The listing builds one solid part. Answer for the finished solid, in the listing's coordinates (mm). A direction names the side the tool comes from. Give positions to 0.01 mm unless a question says otherwise; leave off trailing zeros. Order: outer loops, then holes, each group sorted by start corner. A loop starts at its lowest first (then second) coordinate and runs counter-clockwise, first axis right, second up. Notation, with made-up numbers: (-36, 57) -> (17, 57) arc R28 cw to (17, 75) -> close; hole circle Ø1 at (79, -20.5). An arc over 180 degrees is marked (long way). Answer as a JSON object with one key per item and string values. Group by question number.
```python
from build123d import *

# Parameters (mm, degrees)
F1_DEPTH = 8.89


with BuildPart() as f1:
    # F0 (on Front) → F1 (new body)
    with BuildSketch(Plane.XZ):
        with BuildLine():
            Line((-102.723063, 1.27), (-102.723063, 0))
            Line((-102.723063, 0), (-77.323063, 0))
            Line((-77.323063, 0), (-77.323063, 1.27))
            ThreePointArc((-77.323063, 1.27), (-77.695037, 2.168026), (-78.593063, 2.54))
            Line((-78.593063, 2.54), (-80.879063, 2.54))
            ThreePointArc((-80.879063, 2.54), (-81.058668, 2.614395), (-81.133063, 2.794))
            Line((-81.133063, 2.794), (-81.133063, 5.08))
            ThreePointArc((-81.133063, 5.08), (-81.505037, 5.978026), (-82.403063, 6.35))
            Line((-82.403063, 6.35), (-97.643063, 6.35))
            ThreePointArc((-97.643063, 6.35), (-98.541089, 5.978026), (-98.913063, 5.08))
            Line((-98.913063, 5.08), (-98.913063, 4.318))
            ThreePointArc((-98.913063, 4.318), (-98.541089, 3.419974), (-97.643063, 3.048))
            Line((-97.643063, 3.048), (-95.357063, 3.048))
            ThreePointArc((-95.357063, 3.048), (-95.177458, 3.122395), (-95.103063, 3.302))
            Line((-95.103063, 3.302), (-95.103063, 3.556))
            ThreePointArc((-95.103063, 3.556), (-95.028668, 3.735605), (-94.849063, 3.81))
            Line((-94.849063, 3.81), (-85.197063, 3.81))
            ThreePointArc((-85.197063, 3.81), (-85.017458, 3.735605), (-84.943063, 3.556))
            Line((-84.943063, 3.556), (-84.943063, 2.794))
            ThreePointArc((-84.943063, 2.794), (-85.017458, 2.614395), (-85.197063, 2.54))
            Line((-85.197063, 2.54), (-101.453063, 2.54))
            ThreePointArc((-101.453063, 2.54), (-102.351089, 2.168026), (-102.723063, 1.27))
        make_face()
    extrude(amount=F1_DEPTH)


solid = f1.part
```
(1) Find the intervals of material crossed by line 1 along Z through (x, y) = (-97.75, -0.5); line 2 along Z through (x, y) = (-94.75, -1); line 3 along Z through (x, y) = (-100.75, -4.75), in increasing order. Write a range as [from, to].
(2) Flat-ended cylindrical pins translate along their axes: pin 1 Ø0.6 at (y, z) = (-5.5, 3) entering from -X; pin 2 Ø1.8 at (y, z) = (-6, 4) entering from +X; pin 3 Ø0.6 at (y, z) = (-5, 4.5) entering from -X. Find the tip coordinate at first contact, or state that the pin passes through.
(3) A cutting plane is placed at A-A (x = -86). Determine the outline of the cut face in (y, z), and give its area (3 significant figures).
(4) A cutting plane is placed at B-B (y = -6). Determine the outline of the cut face in (x, z), and give its area (3 significant figures).
(5) Which of the six approach directions +Z, -Z, +X, -X, +Y, -Y give full straight-line access (tool end or side, diameter ignored) to faces 4 (the flat face through (-97, -4, 3.048)), 5 (the flat face through (-90, -4, 3.81)), 6 (the flat face through (-102.723, -4, 1)), 7 (the flat face through (-80, -4, 2.54))?
(6) A cutting plane is placed at D-D (z = 2). Determine the outline of the cut face in (x, y), and give its area (3 significant figures).
(7) A cutting plane is placed at C-C (x = -99.75). Determine the outline of the cut face in (y, z), and give its area (3 significant figures).
(8) For a pull along Z with two mould halves and no side action, classify faces 1 (the cylindrical face through (-98.55, -4.38, 3.43)), 2 (the cylindrical face through (-102.34, -4.38, 2.18)), 3 (the flat face through (-90, 0, 4)) as +Z half, -Z half, draft (parallel to the pull), parting line (faces both ways), or undercut.
Check sheet entries:
{
 "1": {"line 1": "z = [0, 2.54], [3.05, 6.35]", "line 2": "z = [0, 2.54], [3.81, 6.35]", "line 3": "z = [0, 2.54]"},
 "2": {"pin 1": "stops at x = -98.4", "pin 2": "stops at x = -81.13", "pin 3": "stops at x = -98.91"},
 "3": {"outline": "(-8.89, 0) -> (0, 0) -> (0, 2.54) -> (-8.89, 2.54) -> close; (-8.89, 3.81) -> (0, 3.81) -> (0, 6.35) -> (-8.89, 6.35) -> close", "area": "45.2 mm2"},
 "4": {"outline": "(-102.72, 0) -> (-77.32, 0) -> (-77.32, 1.27) arc R1.27 ccw to (-78.59, 2.54) -> (-80.88, 2.54) arc R0.25 cw to (-81.13, 2.79) -> (-81.13, 5.08) arc R1.27 ccw to (-82.4, 6.35) -> (-97.64, 6.35) arc R1.27 ccw to (-98.91, 5.08) -> (-98.91, 4.32) arc R1.27 ccw to (-97.64, 3.05) -> (-95.36, 3.05) arc R0.25 ccw to (-95.1, 3.3) -> (-95.1, 3.56) arc R0.25 cw to (-94.85, 3.81) -> (-85.2, 3.81) arc R0.25 cw to (-84.94, 3.56) -> (-84.94, 2.79) arc R0.25 cw to (-85.2, 2.54) -> (-101.45, 2.54) arc R1.27 ccw to (-102.72, 1.27) -> close", "area": "116 mm2"},
 "5": {"face 4": "-X, +Y, -Y", "face 5": "+Y, -Y", "face 6": "+Z, -Z, -X, +Y, -Y", "face 7": "+Z, +X, +Y, -Y"},
 "6": {"outline": "(-102.49, -8.89) -> (-77.55, -8.89) -> (-77.55, 0) -> (-102.49, 0) -> close", "area": "222 mm2"},
 "7": {"outline": "(-8.89, 0) -> (0, 0) -> (0, 2.54) -> (-8.89, 2.54) -> close", "area": "22.6 mm2"},
 "8": {"face 1": "undercut", "face 2": "+Z half", "face 3": "draft"}
}
